from build123d import *

# Parameters (mm, degrees)
EXTRUDE_2_DEPTH            = 3
SKETCH_4_W                 = 40.9
SKETCH_4_H                 = 2.5
EXTRUDE_3_DEPTH            = 27.7
SKETCH_5_W                 = 40.9
SKETCH_5_H                 = 23
EXTRUDE_4_DEPTH            = 3
CHAMFER_2_SIZE             = 7
SKETCH_8_R                 = 3
CUT_EXTRUDE_3_DEPTH        = 3
CHAMFER_3_SIZE             = 1
CHAMFER_3_OF_MIRROR_1_SIZE = 1
SKETCH_9_W                 = 40.9
SKETCH_9_H                 = 2.5
EXTRUDE_5_DEPTH            = 8


with BuildPart() as part:
    # 스케치3 → 보스-돌출2 (new body)
    with BuildSketch(Plane.XZ.offset(-28.7)):
        with BuildLine():
            Line((-27.85, -6.875), (-27.85, -9))
            Line((-27.85, -9), (-27.85, -13))
            Line((-27.85, -13), (27.85, -13))
            Line((27.85, -13), (27.85, -9))
            Line((27.85, -9), (27.85, -6.875))
            Line((27.85, -6.875), (25.977395688, -6.875))
            ThreePointArc((25.977395688, -6.875), (21.95, -5.65), (25.977395688, -4.425))
            Line((25.977395688, -4.425), (27.85, -4.425))
            Line((27.85, -4.425), (27.85, 4.425))
            Line((27.85, 4.425), (25.977395688, 4.425))
            ThreePointArc((25.977395688, 4.425), (21.95, 5.65), (25.977395688, 6.875))
            Line((25.977395688, 6.875), (27.85, 6.875))
            Line((27.85, 6.875), (27.85, 9))
            ThreePointArc((27.85, 9), (27.557106781, 9.707106781), (26.85, 10))
            Line((26.85, 10), (20.45, 10))
            Line((20.45, 10), (20.45, -10))
            Line((20.45, -10), (20.45, -10.5))
            Line((20.45, -10.5), (-20.45, -10.5))
            Line((-20.45, -10.5), (-20.45, -10))
            Line((-20.45, -10), (-20.45, 10))
            Line((-20.45, 10), (-26.85, 10))
            ThreePointArc((-26.85, 10), (-27.557106781, 9.707106781), (-27.85, 9))
            Line((-27.85, 9), (-27.85, 6.875))
            Line((-27.85, 6.875), (-25.977395688, 6.875))
            ThreePointArc((-25.977395688, 6.875), (-21.95, 5.65), (-25.977395688, 4.425))
            Line((-25.977395688, 4.425), (-27.85, 4.425))
            Line((-27.85, 4.425), (-27.85, -4.425))
            Line((-27.85, -4.425), (-25.977395688, -4.425))
            ThreePointArc((-25.977395688, -4.425), (-21.95, -5.65), (-25.977395688, -6.875))
            Line((-25.977395688, -6.875), (-27.85, -6.875))
        make_face()
    extrude(amount=EXTRUDE_2_DEPTH)

    # 스케치4 → 보스-돌출3 (add)
    with BuildSketch(Plane.XZ.offset(-25.7)):
        with Locations((0, -11.75)):
            Rectangle(SKETCH_4_W, SKETCH_4_H)
    extrude(amount=EXTRUDE_3_DEPTH)

    # 스케치5 → 보스-돌출4 (add)
    with BuildSketch(Plane.XZ.offset(2)):
        with Locations((0, -1.5)):
            Rectangle(SKETCH_5_W, SKETCH_5_H)
    extrude(amount=EXTRUDE_4_DEPTH)

    # 모따기2
    chamfer_2_edges = [part.edges().sort_by_distance(p)[0] for p in [
        (20.45, 25.7, -11.75),
        (-20.45, 25.7, -11.75),
    ]]
    chamfer(chamfer_2_edges, length=CHAMFER_2_SIZE)

    # 스케치8 → 컷-돌출3 (cut)
    with BuildSketch(Plane.XZ.offset(5)):
        with Locations((10.45, 0)):
            Circle(SKETCH_8_R)
    cut_extrude_3 = extrude(amount=-CUT_EXTRUDE_3_DEPTH, mode=Mode.SUBTRACT)

    # 모따기3
    chamfer_3_edges = [part.edges().sort_by_distance(p)[0] for p in [
        (7.45, -5, 0),
    ]]
    chamfer(chamfer_3_edges, length=CHAMFER_3_SIZE)

    # 대칭 복사1: 컷-돌출3 across plane
    add(cut_extrude_3.mirror(Plane(origin=(0, 0, 0), x_dir=(0, 0, 1), z_dir=(1, 0, 0))), mode=Mode.SUBTRACT)

    # 모따기3 of 대칭 복사1
    chamfer_3_of_mirror_1_edges = [part.edges().sort_by_distance(p)[0] for p in [
        (-7.45, -5, 0),
    ]]
    chamfer(chamfer_3_of_mirror_1_edges, length=CHAMFER_3_OF_MIRROR_1_SIZE)

    # 스케치9 → 보스-돌출5 (add)
    with BuildSketch(Plane(origin=(0, 28.7, 0), x_dir=(1, 0, 0), z_dir=(0, 1, 0))):
        with Locations((0, 11.75)):
            Rectangle(SKETCH_9_W, SKETCH_9_H)
    extrude(amount=EXTRUDE_5_DEPTH)


solid = part.part
Could you check a few things on this model? Use its own coordinates, in mm. A direction names the side the tool comes from. Give positions to 0.01 mm unless a question says otherwise; leave off trailing zeros. Order: outer loops, then holes, each group sorted by start corner. A loop starts at its lowest first (then second) coordinate and runs counter-clockwise, first axis right, second up. Notation, with made-up numbers: (31.25, 15) - (60.25, 15) arc R23 cw to (60.25, 39) - close; hole circle Ø4 at (78.5, 60.25). An arc over 180 degrees is marked (long way). One line per item, written item: value. Start each with the question number.
1. For P1, Ø0.9, axis at x = -27.5, y = 26.5, coming from the +Z side; P2, Ø4, axis at x = 3, z = 2.5, coming from the +Y side; P3, Ø6, axis at x = 9, z = -1.5, coming from the -Y side; P4, Ø3.5, axis at x = -23.5, z = -0.5, coming from the -Y side, each with a flat end and sliding along its axis, tell me the tip position at first contact or that it passes through.
2. For faces 1 (the face through (27, 27, -6.875)), 2 (the face through (0, -2, 0)), 3 (the face through (-24, 28.7, -1)), 4 (the face through (-27, 27, 6.875)), which set-ups out of +Z, -Z, +X, -X, +Y, -Y let a thin tool reach every point of the face, with its end or its side?
3. Thinking about a two-plate mould opening in X: for faces 5 (the face through (21.95, 27.22, 5.57)), 6 (the face through (-27.85, 27, 8)), 7 (the face through (27, 27, -4.425)), 8 (the face through (20.45, 27, 0)), which applies, +X half, -X half, draft (parallel to the pull), parting line (faces both ways), or undercut?
4. Imagine slicing it at B-B on x = 10.45. List the corners of the cut face in (y, z) for me, plus the area to 3 significant figures.
5. Imagine slicing it at C-C on x = -24.15. List the corners of the cut face in (y, z) for me, plus the area to 4 significant figures.
6. Imagine slicing it at D-D on z = 0. List the corners of the cut face in (x, y) for me, plus the area to 3 significant figures.
7. Imagine slicing it at A-A on z = -5.65. List the corners of the cut face in (x, y) for me, plus the area to 3 significant figures.
8. If I drill on probe 1 along Z at (x, y) = (-24.15, 27.8); probe 2 along X at (y, z) = (27.2, 5.65); probe 3 along Z at (x, y) = (-10.45, -2.5), over which ranges is the centre line in solid material (lowest first)?
Values:
1. P1: z = 9.98
1. P2: y = -2
1. P3: y = -5
1. P4: y = 25.7
2. face 1: +X, +Y, -Y
2. face 2: +Z, +X, -X, +Y
2. face 3: +Z, -Z, -X, +Y
2. face 4: -X, +Y, -Y
3. face 5: undercut
3. face 6: -X half
3. face 7: draft
3. face 8: undercut
4. outline: (-5, -13) - (36.7, -13) - (36.7, -10.5) - (-2, -10.5) - (-2, -3) - (-4, -3) - (-5, -4) - close; (-5, 4) - (-4, 3) - (-2, 3) - (-2, 10) - (-5, 10) - close
4. area: 147 mm²
5. outline: (22.4, -13) - (28.7, -13) - (28.7, -7.85) - (25.7, -7.85) - (25.7, -10.5) - (22.4, -10.5) - close; (25.7, -3.45) - (28.7, -3.45) - (28.7, 3.45) - (25.7, 3.45) - close; (25.7, 7.85) - (28.7, 7.85) - (28.7, 10) - (25.7, 10) - close
5. area: 50.85 mm²
6. outline: (-27.85, 25.7) - (-20.45, 25.7) - (-20.45, 28.7) - (-27.85, 28.7) - close; (-20.45, -5) - (-14.45, -5) - (-13.45, -4) - (-13.45, -2) - (-20.45, -2) - close; (-7.45, -4) - (-6.45, -5) - (6.45, -5) - (7.45, -4) - (7.45, -2) - (-7.45, -2) - close; (13.45, -4) - (14.45, -5) - (20.45, -5) - (20.45, -2) - (13.45, -2) - close; (20.45, 25.7) - (27.85, 25.7) - (27.85, 28.7) - (20.45, 28.7) - close
6. area: 129 mm²
7. outline: (-21.95, 25.7) - (-20.45, 25.7) - (-20.45, 28.7) - (-21.95, 28.7) - close; (-20.45, -5) - (20.45, -5) - (20.45, -2) - (-20.45, -2) - close; (20.45, 25.7) - (21.95, 25.7) - (21.95, 28.7) - (20.45, 28.7) - close
7. area: 132 mm²
8. probe 1: -13 to -7.85, -3.45 to 3.45, 7.85 to 10
8. probe 2: -21.95 to -20.45, 20.45 to 21.95
8. probe 3: -13 to -3, 3 to 10
